Here's how the part is built. I have some questions about the finished solid (model axes, mm). Face numbers are marked on the shaded views. Round coordinates to 2 decimals unless told otherwise and drop trailing zeros. Loops run counter-clockwise (first coordinate to the right, second up) from the corner with the lowest first, then second, coordinate; pieces in that order, holes last. Notation, with made-up numbers: (44.25, -18.75) - (90.25, -18.75) arc R32 ccw to (90.25, 10.25) - close; hole circle Ø10 at (89, 77.5). An arc over 180 degrees is marked (long way). Answer as a JSON object with one key per item and string values. Group by question number.
1) If we mould it in two halves opening along Y, with no side actions, what happens to the marked faces 1, 2 and 3? For each: pulls with the +Y half, pulls with the -Y half, needs draft (parallel to the pull), parting line crosses it, or undercut.
2) Will this pin go through, and if not, where does the flat tip stop? P1, Ø4, axis at y = 3.5, z = 0.5, coming from the -X side.
3) I want a section at A-A, the plane x = 2.05. Please give me the cut outline in (y, z), then the cut area to 3 significant figures.
4) If I drill on line 1 along Z through (x, y) = (2.8, 0); line 2 along Z through (x, y) = (2.3, 1); line 3 along Y through (x, z) = (1.65, -1), over which ranges is the centre line in solid material (lowest first)? Write a range as [from, to].
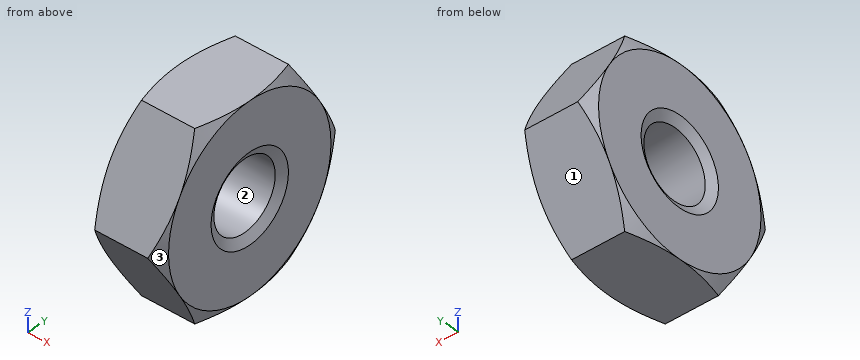
Autodesk Inventor part; units mm, degrees
ref_plane "Work Plane1" through (-10.4473, 0, 0) normal (0, -0.866, -0.5) x (1, 0, 0)
ref_plane "YZ Plane" through (0, 0, 0) normal (1, 0, 0) x (0, 1, 0)
ref_plane "XZ Plane" through (0, 0, 0) normal (0, 1, 0) x (-1, 0, 0)
sketch "Sketch1" plane through (0, 0, 0) normal (1, 0, 0) x (0, 1, 0)
  line L0 (-5.0447, 0) -> (-2.5223, 4.3688)
  line L1 (-2.5223, 4.3688) -> (2.5223, 4.3688)
  line L2 (2.5223, 4.3688) -> (5.0447, 0)
  line L3 (5.0447, 0) -> (2.5223, -4.3688)
  line L4 (2.5223, -4.3688) -> (-2.5223, -4.3688)
  line L5 (-2.5223, -4.3688) -> (-5.0447, 0)
  point P0 (0, 0)
  point P1 (0, 0)
  dimension "d0" = 10.0893
extrude "Body" add sketch "Sketch1" along normal blind 3.302
sketch "Sketch2" plane through (0, 0, 0) normal (0, 0, 1) x (1, 0, 0)
  line L0 (0, 2.5223) -> (0, 5.0447)
  line L1 (0, 5.0447) -> (3.302, 5.0447)
  line L2 (3.302, 2.5223) -> (3.302, 5.0447)
  line L3 (-0.6604, 0) -> (3.9624, 0)
  line L4 (0.3902, 5.0447) -> (0, 4.3688)
  line L5 (2.9118, 5.0447) -> (3.302, 4.3688)
  dimension "d3" = 30
  dimension "d4" = 30
  dimension "d5" = 8.7376
  dimension "d6" = 8.7376
revolve "Chamfer1" cut sketch "Sketch2" angle 360 about axis through (-10, 0, 0) along (1, 0, 0)
sketch "Sketch3" plane through (3.302, 0, 0) normal (1, 0, 0) x (0, 0, -1)
  arc A0 (-2.1844, -3.7835) -> (2.1844, -3.7835) centre (0, 0) ccw
hole "Thread" at (3.302, 0, 0) direction (-1, 0, 0) diameter 3.302 end through all
chamfer "Chamfer2" distance 0.4296 angle 30 1 edges at (3.302, 0, 1.651) measured on face at (3.302, 3.4429, -0.0663)
chamfer "Chamfer3" distance 0.4296 angle 30 1 edges at (0, 0, 1.651) measured on face at (0, 3.4429, -0.0663)
ref_plane "Work Plane1" through (-10.4473, 0, 0) normal (0, -0.866, -0.5) x (1, 0, 0)
equation "\"d0\" = 1.1547 * SW"
equation "\"d1\" = KOH"
equation "\"d3\" = ANG1"
equation "\"d4\" = ANG2"
equation "\"d5\" = SW0"
equation "\"d6\" = SW01"
equation "\"d8\" = -0.5 * GD1 + 0.5 * NND"
equation "\"d40\" = -0.5 * GD1 + 0.5 * NND"
equation "\"d10\" = -0.5 * GD1 + 0.5 * NND"
equation "\"d41\" = -0.5 * GD1 + 0.5 * NND"
equation "\"ANG1\" = 30deg"
equation "\"ANG2\" = 30deg"
equation "\"NND\" = 4.1656"
equation "\"KOH\" = 3.302"
equation "\"SW\" = 8.7376"
equation "\"SW0\" = SW"
equation "\"SW01\" = SW"
equation "\"THREADDIA\" = 4.1656"
equation "\"TOA\" = 30deg"
equation "\"E0\" = 1.155 * SW"
properties part number "ANSI B18.2.2 - 8 - 32, HMSNI" material "Steel, Mild"
Outcome:
{
 "1": {"face 1": "pulls with the +Y half", "face 2": "undercut", "face 3": "pulls with the -Y half"},
 "2": {"P1": "x = 0"},
 "3": {"outline": "(-5.04, 0) - (-2.52, -4.37) - (2.52, -4.37) - (5.04, 0) - (2.52, 4.37) - (-2.52, 4.37) - close; hole circle Ø3.3 at (0, 0)", "area": "57.6 mm^2"},
 "4": {"line 1": "[-4.37, -1.65], [1.65, 4.37]", "line 2": "[-4.37, -1.31], [1.31, 4.37]", "line 3": "[-4.47, -1.31], [1.31, 4.47]"}
}
